```python
from build123d import *

# Parameters (mm, degrees)
F3_W     = 63.5
F3_H     = 19.05
F3_R     = 3.175
F3_W_2   = 19.05
F4_DEPTH = 19.05


with BuildPart() as f4:
    # F3 (on Front) → F4 (new body)
    with BuildSketch(Plane.XZ):
        Rectangle(F3_W, F3_H)
        with Locations((-22.225, 0)):
            Circle(F3_R, mode=Mode.SUBTRACT)
        with Locations((22.225, 0)):
            Circle(F3_R, mode=Mode.SUBTRACT)
        with Locations((41.275, 0)):
            Rectangle(F3_W_2, F3_H)
        with Locations((-41.275, 0)):
            Rectangle(F3_W_2, F3_H)
    extrude(amount=F4_DEPTH)


solid = f4.part
```
Geometry check sheet. Reference: the model listing, model coordinates, mm. Round coordinates to 2 decimals unless told otherwise and drop trailing zeros. Loops run counter-clockwise (first coordinate to the right, second up) from the corner with the lowest first, then second, coordinate; pieces in that order, holes last. Notation, with made-up numbers: (-32, 32) - (19, 32) arc R16 cw to (19, 47) - close; hole circle Ø6 at (83.25, 37). An arc over 180 degrees is marked (long way). Write each question's results on one line, items separated by ' | '. Start each with the question number.
Q1. Cross-section at B-B on y = -5.75. Enter the section's corners in (x, z) (3 decimals).
Q2. Cross-section at C-C on x = 24. Enter the section's corners in (y, z) (3 decimals).
Q3. Release check for a two-part mould opening along Z. For faces 1 (the flat face through (50.8, -9, 0)), 2 (the cylindrical face through (-19.197, -9.392, 0.954)), 3 (the cylindrical face through (25.253, -9.392, 0.954)), 4 (the flat face through (-1, -9, -9.525)) record: +Z half, -Z half, draft (parallel to the pull), parting line (faces both ways), or undercut.
Q4. Cross-section at A-A on z = 0. Enter the section's corners in (x, y), and give its area (3 significant figures).
Q5. Thickness scan on line 1 (X direction, y = -14.5, z = -2); line 2 (X direction, y = -13.25, z = 0.75); line 3 (Z direction, x = 24, y = -10) (3 decimals). Record the ranges inside material, lowest first. Write a range as [from, to].
Answers below:
1) outline: (-50.8, -9.525) - (50.8, -9.525) - (50.8, 9.525) - (-50.8, 9.525) - close; hole circle Ø6.35 at (-22.225, 0); hole circle Ø6.35 at (22.225, 0)
2) outline: (-19.05, -9.525) - (0, -9.525) - (0, -2.632) - (-19.05, -2.632) - close; (-19.05, 2.632) - (0, 2.632) - (0, 9.525) - (-19.05, 9.525) - close
3) face 1: draft | face 2: undercut | face 3: undercut | face 4: -Z half
4) outline: (-50.8, -19.05) - (-25.4, -19.05) - (-25.4, 0) - (-50.8, 0) - close; (-19.05, -19.05) - (19.05, -19.05) - (19.05, 0) - (-19.05, 0) - close; (25.4, -19.05) - (50.8, -19.05) - (50.8, 0) - (25.4, 0) - close | area: 1,690 mm²
5) line 1: x = [-50.8, -24.69], [-19.76, 19.76], [24.69, 50.8] | line 2: x = [-50.8, -25.31], [-19.14, 19.14], [25.31, 50.8] | line 3: z = [-9.525, -2.632], [2.632, 9.525]
